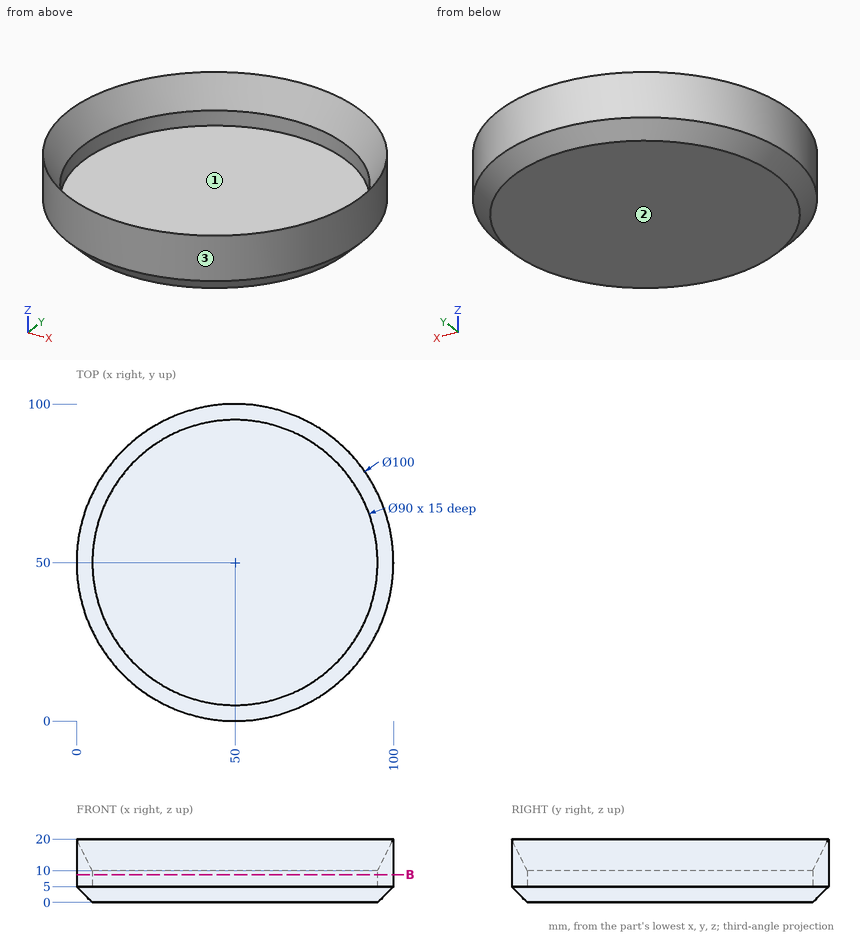
Geometry: see drawing. Coordinates: mm, zero at the bounding-box minimum. Coordinates: 2 decimals unless noted, no trailing zeros. Loops run counter-clockwise (first coordinate to the right, second up) from the corner with the lowest first, then second, coordinate; pieces in that order, holes last. Notation, with made-up numbers: (-23.75, 13) -> (3.25, 13) arc R27 cw to (3.25, 33) -> close; hole circle Ø8 at (-9, -38.5). An arc over 180 degrees is marked (long way). Use a Markdown table: item, result.
1) Contact query for flat-ended pins moving along their axis: pin 1 (5 mm diameter, centred on x = 50, y = 73, fed in from -Z); pin 2 (4 mm diameter, centred on y = 54.5, z = 8.5, fed in from -X); pin 3 (12 mm diameter, centred on y = 18.5, z = 4, fed in from +X); pin 4 (3 mm diameter, centred on x = 75.5, y = 10.5, fed in from -Z). Output: stop coordinate, or through.
Results found:
| item | result |
|---|---|
| pin 1 | stops at z = 0 |
| pin 2 | stops at x = 0.06 |
| pin 3 | stops at x = 92.96 |
| pin 4 | stops at z = 0.52 |
2) Pull-direction query (X, two-part tool) for the marked faces 1, 2 and 3; classes: released by +X, released by -X, zero draft, split by the parting line, or undercut.
Results found:
| item | result |
|---|---|
| face 1 | undercut |
| face 2 | zero draft |
| face 3 | split by the parting line |
3) Cut plane B-B (z = 8.75). Return the cut outline in (x, y), then the cut area to 3 significant figures.
Results found:
| item | result |
|---|---|
| outline | circle Ø100 at (50, 50); hole circle Ø90 at (50, 50) |
| area | 1,490 mm2 |
4) Material intervals for line 1 along Y through (x, z) = (50, 6.35); line 2 along Z through (x, y) = (59, 49); line 3 along X through (y, z) = (57, 11.5), sorted ascending. Write a range as from..to.
Results found:
| item | result |
|---|---|
| line 1 | y = 0..5, 95..100 |
| line 2 | z = 0..5 |
| line 3 | x = 0.49..4.79, 95.21..99.51 |
